Part model, mm, in its own coordinate system. Give positions to 0.01 mm unless a question says otherwise; leave off trailing zeros. Write each loop counter-clockwise with the first axis right and the second up, starting at its lowest first coordinate (ties: lowest second). Pieces come first, ordered by that corner, then holes. Notation, with made-up numbers: M 67,14 L 90,14 A27 cw 90,36 Z; hole C 23,33.5 d5. An arc over 180 degrees is marked long. Use a Markdown table: item, result.
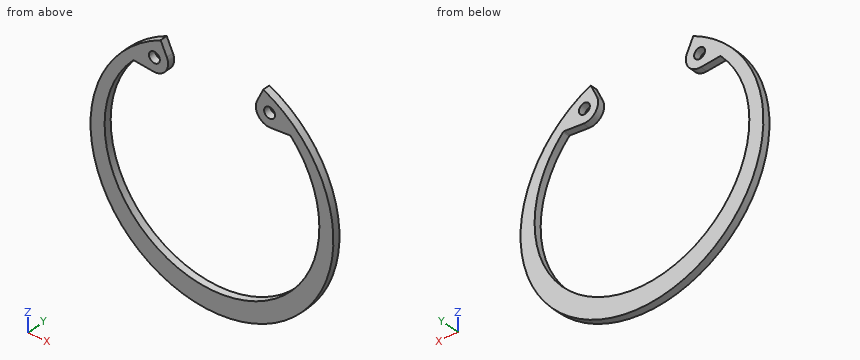
```python
from build123d import *

# Parameters (mm, degrees)
SKETCH2_R      = 1.1811
EXTRUDE1_DEPTH = 1.5748
FILLET1_R      = 0.254


with BuildPart() as part:
    # Sketch2 → Extrude1 (new body)
    with BuildSketch(Plane(origin=(0, 0, 0), x_dir=(1, 0, 0), z_dir=(0, 1, 0))):
        with BuildLine():
            Line((11.120945987, -23.848945631), (9.784734318, -20.98343046))
            ThreePointArc((9.784734318, -20.98343046), (10.043743754, -18.022939056), (12.737109235, -16.767002106))
            Line((12.737109235, -16.767002106), (17.019050922, -17.141623461))
            ThreePointArc((17.019050922, -17.141623461), (0, 21.9964), (-17.019050922, -17.141623461))
            Line((-17.019050922, -17.141623461), (-12.737109235, -16.767002106))
            ThreePointArc((-12.737109235, -16.767002106), (-10.043743754, -18.022939056), (-9.784734318, -20.98343046))
            Line((-9.784734318, -20.98343046), (-11.120945987, -23.848945631))
            ThreePointArc((-11.120945987, -23.848945631), (0, 26.3144), (11.120945987, -23.848945631))
        make_face()
        with Locations(Location((12.478099799, -19.727493509, 0), (0, 0, 270))):
            Circle(SKETCH2_R, mode=Mode.SUBTRACT)
        with Locations(Location((-12.478099799, -19.727493509, 0), (0, 0, 270))):
            Circle(SKETCH2_R, mode=Mode.SUBTRACT)
    extrude(amount=-EXTRUDE1_DEPTH)

    # Fillet1
    fillet1_edges = [part.edges().sort_by_distance(p)[0] for p in [
        (17.019050922, -0.7874, 17.141623461),
        (-17.019050922, -0.7874, 17.141623461),
    ]]
    fillet(fillet1_edges, radius=FILLET1_R)


solid = part.part
```
1. Cut at B-B, the plane y = -1.25. Give the cut face in (x, z), then the cut area to 3 significant figures.
Findings below:
| item | result |
|---|---|
| outline | M -17.1,17.05 A0.25 cw -16.9,17.13 L -12.74,16.77 A2.97 ccw -9.78,20.98 L -11.12,23.85 A26.31 ccw long 11.12,23.85 L 9.78,20.98 A2.97 ccw 12.74,16.77 L 16.9,17.13 A0.25 cw 17.1,17.05 A23.27 cw long Z; hole C -12.48,19.73 d2.36; hole C 12.48,19.73 d2.36 |
| area | 470 mm2 |
2. Cut at D-D, the plane z = 0. Give the cut face in (x, y), then the cut area to 3 significant figures.
Findings below:
| item | result |
|---|---|
| outline | M -26.31,-1.57 L -23.23,-1.57 L -23.23,0 L -26.31,0 Z; M 23.23,-1.57 L 26.31,-1.57 L 26.31,0 L 23.23,0 Z |
| area | 9.70 mm2 |
3. Cut at C-C, the plane x = 0. Give the cut face in (y, z).
Findings below:
| item | result |
|---|---|
| outline | M -1.57,-26.31 L 0,-26.31 L 0,-22 L -1.57,-22 Z |
4. Cut at A-A, the plane z = -9.5. Give the cut face in (x, y), then the cut area to 3 significant figures.
Findings below:
| item | result |
|---|---|
| outline | M -24.54,-1.57 L -20.63,-1.57 L -20.63,0 L -24.54,0 Z; M 20.63,-1.57 L 24.54,-1.57 L 24.54,0 L 20.63,0 Z |
| area | 12.3 mm2 |
5. Drill centre lines: L1, parallel to Z at x = 13.5, y = -0.8; L2, parallel to X at y = -0.95, z = 20; L3, parallel to Z at x = 0, y = -0.85. Where is each one in solid material? Low to high.
Findings below:
| item | result |
|---|---|
| L1 | -22.59 to -17.68, 16.83 to 19.14, 20.32 to 22.59 |
| L2 | -17.1 to -13.63, -11.33 to -9.52, 9.52 to 11.33, 13.63 to 17.1 |
| L3 | -26.31 to -22 |
